Design review of the part built by this model. Coordinates are the model's own, in mm. A direction names the side the tool comes from. Coordinates: 2 decimals unless noted, no trailing zeros. Order: outer loops, then holes, each group sorted by start corner. A loop starts at its lowest first (then second) coordinate and runs counter-clockwise, first axis right, second up. Notation, with made-up numbers: M -26.75,-2 L -8.75,-2 A28 cw -8.75,33 Z; hole C 86.5,73.25 d2. An arc over 180 degrees is marked long. Answer in a Markdown table with one row per item.
from build123d import *

# Parameters (mm, degrees)
F0_W     = 107.8754812479
F0_H     = 26.1090872809
F1_DEPTH = 12.7
F2_DEPTH = 12.7
F3_R     = 11.2223896829
F4_DEPTH = 177.8
F6_DEPTH = 482.6
F7_SIZE2 = 11.1616915599
F7_SIZE  = 41.656


with BuildPart() as f1:
    # F0 (on Front) → F1 (new body)
    with BuildSketch(Plane.XZ):
        with Locations((0.7920116186, 0.3961385228)):
            Rectangle(F0_W, F0_H)
    extrude(amount=F1_DEPTH)

    # F2 (add): a face of the model
    f2_faces = [f1.faces().sort_by_distance(p)[0] for p in [
        (0.7920116186, 0, 0.3961385228),
    ]]
    extrude(f2_faces, amount=F2_DEPTH)

    # F3 (on face) → F4 (join)
    with BuildSketch(Plane(origin=(0, 0, -12.6584051177), x_dir=(1, 0, 0), z_dir=(0, 0, -1))):
        Circle(F3_R)
    extrude(amount=F4_DEPTH)

    # F5 (on face) → F6 (join)
    with BuildSketch(Plane.XY.offset(13.4506821632)):
        Polygon((36.2057685852, 0), (0, 11.8748378009), (-36.2340435386, 0), (0, -11.7327794433), align=None)
    extrude(amount=F6_DEPTH)

    # F7
    f7_edges = [f1.edges().sort_by_distance(p)[0] for p in [
        (-18.117022, -5.86639, 496.050682),
        (18.102884, -5.86639, 496.050682),
        (18.102884, 5.937419, 496.050682),
        (-18.117022, 5.937419, 496.050682),
    ]]
    chamfer(f7_edges, length=F7_SIZE, length2=F7_SIZE2)


solid = f1.part
(1) Add section C-C, the plane z = 110. Give the boundary of the cut face in (x, y), and give its area (3 significant figures).
Return value:
| item | result |
|---|---|
| outline | M -36.23,0 L 0,-11.73 L 36.21,0 L 0,11.87 Z |
| area | 855 mm2 |
(2) Add section A-A, the plane x = 22. Give the boundary of the cut face in (y, z), and give its area (3 significant figures).
Return value:
| item | result |
|---|---|
| outline | M -12.7,-12.66 L 12.7,-12.66 L 12.7,13.45 L 4.66,13.45 L 4.66,454.39 L 0.03,470.83 L -4.6,454.39 L -4.6,13.45 L -12.7,13.45 Z |
| area | 4,820 mm2 |
(3) Insertion check: pin 1 Ø3 at (x, z) = (15, 108.5) entering from -Y; pin 2 Ø1 at (x, y) = (-37.5, 9.5) entering from +Z; pin 3 Ø4 at (x, y) = (-36.5, -1.5) entering from +Z. Each pin has a flat end and moves straight along its axis. Give the tip position at first contact, or say it passes through.
Return value:
| item | result |
|---|---|
| pin 1 | stops at y = -7.36 |
| pin 2 | stops at z = 13.45 |
| pin 3 | stops at z = 455.61 |
(4) Add section D-D, the plane x = -25. Give the boundary of the cut face in (y, z).
Return value:
| item | result |
|---|---|
| outline | M -12.7,-12.66 L 12.7,-12.66 L 12.7,13.45 L 3.68,13.45 L 3.68,454.39 L 0.02,467.38 L -3.64,454.39 L -3.64,13.45 L -12.7,13.45 Z |
(5) For line 1 along Z through (x, y) = (6, -11); line 2 along X through (y, z) = (1.25, -68); line 3 along Y through (x, z) = (23, 321), list the stretches that pass through material, from the lowest coordinate up. Write a range as from..to.
Return value:
| item | result |
|---|---|
| line 1 | z = -12.66..13.45 |
| line 2 | x = -11.15..11.15 |
| line 3 | y = -4.28..4.33 |
(6) Add section B-B, the plane y = -5. Give the boundary of the cut face in (x, z).
Return value:
| item | result |
|---|---|
| outline | M -53.15,-12.66 L -10.05,-12.66 L -10.05,-190.46 L 10.05,-190.46 L 10.05,-12.66 L 54.73,-12.66 L 54.73,13.45 L 20.78,13.45 L 20.78,454.39 L 0,478.3 L -20.79,454.39 L -20.79,13.45 L -53.15,13.45 Z |
(7) For faces 1 (the flat face through (-18.371, -5.784, 230.836)), 2 (the cylindrical face through (-2.433, 10.956, -100.314)), 3 (the flat face through (-17.86, 6.02, 230.84)), 4 (the flat face through (-12, -9, 13.451)), list the 3-axis set-ups (+Z, -Z, +X, -X, +Y, -Y) from which the entire face can be reached by the end or side of a thin tool; tool diameter is ignored.
Return value:
| item | result |
|---|---|
| face 1 | +Z, -X, -Y |
| face 2 | -Z |
| face 3 | +Z, -X, +Y |
| face 4 | +Z |
